Check sheet for the modelled part. Datum: model origin and axes. Units: mm. A direction names the side the tool comes from. Give positions to 0.01 mm unless a question says otherwise; leave off trailing zeros. Write each loop counter-clockwise with the first axis right and the second up, starting at its lowest first coordinate (ties: lowest second). Pieces come first, ordered by that corner, then holes. Notation, with made-up numbers: (-36, 70) -> (-30, 70) arc R14 ccw to (-30, 79) -> close; hole circle Ø8 at (36.5, 82.25). An arc over 180 degrees is marked (long way). Answer as a JSON object with one key per item and string values.
from build123d import *

# Parameters (mm, degrees)
F0_W      = 68
F0_H      = 53
F1_DEPTH  = 26
F2_W      = 63.165789
F2_H      = 48.126318
F3_DEPTH  = 24
F4_W      = 20.754472
F4_H      = 47.825529
F5_DEPTH  = 25.4
F6_W      = 62.564209
F6_H      = 21.055263
F7_DEPTH  = 25.4
F8_W      = 62.865002
F8_H      = 21.055264
F9_DEPTH  = 25.4
F10_W     = 21.055262
F10_H     = 48.126317
F11_DEPTH = 25.4


with BuildPart() as f1:
    # F0 (on Front) → F1 (new body)
    with BuildSketch(Plane.XZ):
        with Locations((-9.898553, 29.29739)):
            Rectangle(F0_W, F0_H)
    extrude(amount=F1_DEPTH)

    # F2 (on face) → F3 (cut)
    with BuildSketch(Plane.XZ.offset(26)):
        with Locations((-10.076449, 29.326975)):
            Rectangle(F2_W, F2_H)
    extrude(amount=-F3_DEPTH, mode=Mode.SUBTRACT)

    # F4 (on face) → F5 (cut)
    with BuildSketch(Plane.YZ.offset(24.101447)):
        with Locations((-12.933949, 29.477369)):
            Rectangle(F4_W, F4_H)
    extrude(amount=-F5_DEPTH, mode=Mode.SUBTRACT)

    # F6 (on face) → F7 (cut)
    with BuildSketch(Plane(origin=(0, 0, 2.79739), x_dir=(1, 0, 0), z_dir=(0, 0, -1))):
        with Locations((-10.076449, 13.084342)):
            Rectangle(F6_W, F6_H)
    extrude(amount=-F7_DEPTH, mode=Mode.SUBTRACT)

    # F8 (on face) → F9 (cut)
    with BuildSketch(Plane.XY.offset(55.79739)):
        with Locations((-10.226843, -12.783553)):
            Rectangle(F8_W, F8_H)
    extrude(amount=-F9_DEPTH, mode=Mode.SUBTRACT)

    # F10 (on face) → F11 (cut)
    with BuildSketch(Plane(origin=(-43.898553, 0, 0), x_dir=(0, -1, 0), z_dir=(-1, 0, 0))):
        with Locations((12.783554, 29.627764)):
            Rectangle(F10_W, F10_H)
    extrude(amount=-F11_DEPTH, mode=Mode.SUBTRACT)


solid = f1.part
1. Scan lines: L1, parallel to Y at x = 14.5, z = 5; L2, parallel to Y at x = -28, z = 19.5. Record each from-to range of solid material in increasing order. Write a range as [from, to].
Determined:
{"L1": "[-26, -23.61], [-2.56, 0]", "L2": "[-2, 0]"}
2. Sectioned sample at B-B, the plane z = 51.5. Enter the section's corners in (x, y), plus the area to 3 significant figures.
Determined:
{"outline": "(-43.9, -26) -> (-41.66, -26) -> (-41.66, -23.31) -> (-43.9, -23.31) -> close; (-43.9, -2.26) -> (-41.66, -2.26) -> (-41.66, -2) -> (21.51, -2) -> (21.51, -2.56) -> (24.1, -2.56) -> (24.1, 0) -> (-43.9, 0) -> close; (21.51, -26) -> (24.1, -26) -> (24.1, -23.31) -> (21.51, -23.31) -> close", "area": "151 mm^2"}
3. Mould release check, pull along Y, two halves, no side actions. Record for faces 5 (the face through (21.506, -24, 27)), 6 (the face through (-43, -13, 5.565)), 7 (the face through (-13, -26, 4)): released by +Y, released by -Y, zero draft, split by the parting line, or undercut.
Determined:
{"face 5": "zero draft", "face 6": "undercut", "face 7": "released by -Y"}
4. Sectioned sample at A-A, the plane y = -8. Enter the section's corners in (x, z).
Determined:
{"outline": "(-43.9, 2.8) -> (-41.36, 2.8) -> (-41.36, 5.26) -> (-41.66, 5.26) -> (-41.66, 5.56) -> (-43.9, 5.56) -> close; (-43.9, 53.69) -> (-41.66, 53.69) -> (-41.66, 55.8) -> (-43.9, 55.8) -> close; (21.21, 2.8) -> (24.1, 2.8) -> (24.1, 5.56) -> (21.51, 5.56) -> (21.51, 5.26) -> (21.21, 5.26) -> close; (21.21, 53.39) -> (24.1, 53.39) -> (24.1, 55.8) -> (21.21, 55.8) -> close"}
5. Go/stop test with a flat-tipped pin: P1, Ø12.5, axis at x = -23, z = 39.5, coming from the -Y side. Record where the tip stops, or that it passes through.
Determined:
{"P1": "y = -2"}
6. Sectioned sample at C-C, the plane x = -29.5. Enter the section's corners in (y, z).
Determined:
{"outline": "(-26, 2.8) -> (-23.61, 2.8) -> (-23.61, 5.26) -> (-26, 5.26) -> close; (-26, 53.39) -> (-23.31, 53.39) -> (-23.31, 55.8) -> (-26, 55.8) -> close; (-2.56, 2.8) -> (0, 2.8) -> (0, 55.8) -> (-2.26, 55.8) -> (-2.26, 53.39) -> (-2, 53.39) -> (-2, 5.26) -> (-2.56, 5.26) -> close"}
7. Access from +Z, -Z, +X, -X, +Y, -Y to the whole of each face (thin tool, end or side, straight path). Record for faces 1 (the face through (-43, -2.256, 29)), 2 (the face through (-10, -2.256, 54)), 3 (the face through (-11, -2, 30)), 4 (the face through (23, -23.311, 29)).
Determined:
{"face 1": "-X", "face 2": "+Z", "face 3": "-Y", "face 4": "+X, -X"}
